from build123d import *

# Parameters (mm, degrees)
F0_W      = 140
F0_H      = 160
F1_DEPTH  = 3
F2_W      = 140
F2_H      = 160
F2_W_2    = 134
F2_H_2    = 154
F3_DEPTH  = 50
F4_W      = 170
F4_H      = 200
F4_W_2    = 140
F4_H_2    = 160
F4_W_3    = 134
F4_H_3    = 154
F5_DEPTH  = 3
F8_R      = 1.5
F10_DEPTH = 170
F6_W      = 15
F6_H      = 7
F6_H_2    = 3
F6_W_2    = 8
F6_H_3    = 5
F11_DEPTH = 25
F7_W      = 8
F7_H      = 5
F7_H_2    = 3
F12_DEPTH = 25
F14_DEPTH = 200
F16_DEPTH = 200
F18_DEPTH = 170


with BuildPart() as f1:
    # F0 (on Top) → F1 (new body)
    with BuildSketch(Plane.XY):
        Rectangle(F0_W, F0_H)
    extrude(amount=F1_DEPTH)

    # F2 (on face) → F3 (join)
    with BuildSketch(Plane.XY.offset(3)):
        Rectangle(F2_W, F2_H)
        Rectangle(F2_W_2, F2_H_2, mode=Mode.SUBTRACT)
    extrude(amount=F3_DEPTH)

    # F4 (on face) → F5 (join)
    with BuildSketch(Plane.XY.offset(53)):
        Rectangle(F4_W, F4_H)
        Rectangle(F4_W_2, F4_H_2, mode=Mode.SUBTRACT)
        Rectangle(F4_W_2, F4_H_2)
        Rectangle(F4_W_3, F4_H_3, mode=Mode.SUBTRACT)
    extrude(amount=F5_DEPTH)

    # F8
    f8_edges = [f1.edges().sort_by_distance(p)[0] for p in [
        (-70, 0, 0),
        (0, -80, 0),
        (70, 0, 0),
        (0, 80, 0),
        (-70, 80, 26.5),
        (70, 80, 26.5),
        (-70, -80, 26.5),
        (70, -80, 26.5),
    ]]
    fillet(f8_edges, radius=F8_R)

    # F9 (on face) → F10 (join, through all)
    with BuildSketch(Plane(origin=(-85, 0, 0), x_dir=(0, -1, 0), z_dir=(-1, 0, 0))):
        Polygon((-80, 53), (-100, 53), (-80, 36.92748), align=None)
        Polygon((100, 53), (80, 53), (80, 36.92748), align=None)
    extrude(amount=-F10_DEPTH)

    # F6 (on face) → F11 (cut)
    with BuildSketch(Plane(origin=(0, 100, 0), x_dir=(-1, 0, 0), z_dir=(0, 1, 0))):
        with Locations((-56.994275, 49.5)):
            Rectangle(F6_W, F6_H)
        with Locations((-56.994275, 54.5)):
            Rectangle(F6_W, F6_H_2)
        with Locations((54.582062, 50.5)):
            Rectangle(F6_W_2, F6_H_3)
        with Locations((54.582062, 54.5)):
            Rectangle(F6_W_2, F6_H_2)
    extrude(amount=-F11_DEPTH, mode=Mode.SUBTRACT)

    # F7 (on face) → F12 (cut)
    with BuildSketch(Plane.XZ.offset(100)):
        with Locations((57.574429, 50.5)):
            Rectangle(F7_W, F7_H)
        with Locations((57.574429, 54.5)):
            Rectangle(F7_W, F7_H_2)
    extrude(amount=-F12_DEPTH, mode=Mode.SUBTRACT)

    # F13 (on face) → F14 (join, through all)
    with BuildSketch(Plane(origin=(0, 100, 0), x_dir=(-1, 0, 0), z_dir=(0, 1, 0))):
        Polygon((-70, 53), (-85, 53), (-70, 36.92748), align=None)
        Polygon((70, 53), (70, 36.92748), (85, 53), align=None)
    extrude(amount=-F14_DEPTH)

    # F15 (on face) → F16 (cut, through all)
    with BuildSketch(Plane(origin=(0, 100, 0), x_dir=(-1, 0, 0), z_dir=(0, 1, 0))):
        Polygon((-70, 36.92748), (-85, 53), (-85, 36.92748), align=None)
        Polygon((85, 36.92748), (85, 53), (70, 36.92748), align=None)
    extrude(amount=-F16_DEPTH, mode=Mode.SUBTRACT)

    # F17 (on face) → F18 (cut, through all)
    with BuildSketch(Plane.YZ.offset(85)):
        Polygon((-80, 36.92748), (-100, 53), (-100, 36.92748), align=None)
        Polygon((100, 36.92748), (100, 53), (80, 36.92748), align=None)
    extrude(amount=-F18_DEPTH, mode=Mode.SUBTRACT)


solid = f1.part
Build history of the part. All positions in model axes, mm. A direction names the side the tool comes from. Coordinates: 2 decimals unless noted, no trailing zeros. Order: outer loops, then holes, each group sorted by start corner. A loop starts at its lowest first (then second) coordinate and runs counter-clockwise, first axis right, second up. Notation, with made-up numbers: (14.5, 25.5) -> (52.5, 25.5) arc R35 ccw to (52.5, 62.5) -> close; hole circle Ø1 at (31, -4.5). An arc over 180 degrees is marked (long way). One line per item, written item: value.
(1) Drop flat-ended pins along their axis: pin 1 Ø8 at (y, z) = (-49, 45.5) entering from -X; pin 2 Ø16 at (y, z) = (-23, 17.5) entering from -X; pin 3 Ø1.2 at (x, y) = (69, 79.5) entering from -Z. Give the stop position or say it passes through.
Checked values:
pin 1: x = -81.73
pin 2: x = -70
pin 3: z = 0.09
(2) Probe line 1 (Y direction, x = 27.5, z = 18); line 2 (X direction, y = 48, z = 35); line 3 (X direction, y = 50, z = 41.5). List the from-to ranges inside material, lowest first. Write a range as [from, to].
Checked values:
line 1: [-80, -77], [77, 80]
line 2: [-70, -67], [67, 70]
line 3: [-74.27, -67], [67, 74.27]
(3) Mould opens along Y. For faces 1 (the flat face through (-1.19, 90.14, 45.076)), 2 (the flat face through (-67, -1, 29)), 3 (the flat face through (1.19, -89.86, 44.85)), 4 (the flat face through (61.574, -89, 52)) say: pulls with the +Y half, pulls with the -Y half, needs draft (parallel to the pull), parting line crosses it, or undercut.
Checked values:
face 1: pulls with the +Y half
face 2: undercut
face 3: pulls with the -Y half
face 4: needs draft
(4) Tool access for faces 5 (the flat face through (-70, -1, 19)), 6 (the flat face through (49.494, 86, 51)), 7 (the flat face through (53.574, -89, 52)): list every direction of +Z, -Z, +X, -X, +Y, -Y with a clear straight run to the whole face (end or side of a thin tool).
Checked values:
face 5: -Z, -X, +Y, -Y
face 6: +Z, +Y
face 7: +Z, +Y, -Y
(5) Slice it at B-B, the plane y = 22. List the corners of the cut face in (x, z).
Checked values:
outline: (-85, 53) -> (-70, 36.93) -> (-70, 1.5) arc R1.5 ccw to (-68.5, 0) -> (68.5, 0) arc R1.5 ccw to (70, 1.5) -> (70, 36.93) -> (85, 53) -> (85, 56) -> (67, 56) -> (67, 3) -> (-67, 3) -> (-67, 56) -> (-85, 56) -> close
(6) Slice it at A-A, the plane z = 27. List the corners of the cut face in (x, y).
Checked values:
outline: (-70, -78.5) arc R1.5 ccw to (-68.5, -80) -> (68.5, -80) arc R1.5 ccw to (70, -78.5) -> (70, 78.5) arc R1.5 ccw to (68.5, 80) -> (-68.5, 80) arc R1.5 ccw to (-70, 78.5) -> close; hole (-67, -77) -> (67, -77) -> (67, 77) -> (-67, 77) -> close
(7) Slice it at C-C, the plane x = 31.5. List the corners of the cut face in (y, z), plus the area to 3 significant figures.
Checked values:
outline: (-100, 53) -> (-80, 36.93) -> (-80, 1.5) arc R1.5 ccw to (-78.5, 0) -> (78.5, 0) arc R1.5 ccw to (80, 1.5) -> (80, 36.93) -> (100, 53) -> (100, 56) -> (77, 56) -> (77, 3) -> (-77, 3) -> (-77, 56) -> (-100, 56) -> close
area: 1,240 mm2
